from build123d import *

# Parameters (mm, degrees)
SKETCH_1_R      = 18.5
SKETCH_1_R_2    = 5
SKETCH_1_R_3    = 2
SKETCH_1_R_4    = 2.08
EXTRUDE_1_DEPTH = 2


with BuildPart() as part:
    # 草图1 → 凸台-拉伸1 (new body)
    with BuildSketch(Plane.XY):
        Circle(SKETCH_1_R)
        Circle(SKETCH_1_R_2, mode=Mode.SUBTRACT)
        with Locations((0, 15)):
            Circle(SKETCH_1_R_3, mode=Mode.SUBTRACT)
        with Locations((12.990381057, -7.5)):
            Circle(SKETCH_1_R_3, mode=Mode.SUBTRACT)
        with Locations((-12.990381057, -7.5)):
            Circle(SKETCH_1_R_3, mode=Mode.SUBTRACT)
        with Locations((-12.36258754, 7.137543244)):
            Circle(SKETCH_1_R_4, mode=Mode.SUBTRACT)
        with Locations((12.36258754, 7.137543244)):
            Circle(SKETCH_1_R_4, mode=Mode.SUBTRACT)
        with Locations((0, -14.275086489)):
            Circle(SKETCH_1_R_4, mode=Mode.SUBTRACT)
    extrude(amount=EXTRUDE_1_DEPTH)


solid = part.part
Geometry: final body of the model. Coordinates: model frame, mm. Give positions to 0.01 mm unless a question says otherwise; leave off trailing zeros. Order: outer loops, then holes, each group sorted by start corner. A loop starts at its lowest first (then second) coordinate and runs counter-clockwise, first axis right, second up. Notation, with made-up numbers: (65.25, 26) -> (84.25, 26) arc R28 cw to (84.25, 64) -> close; hole circle Ø8 at (71, 83). An arc over 180 degrees is marked (long way). Answer as a JSON object with one key per item and string values.
Q1. Section D-D (y = -6). Output: boundary loops of the cut face in (x, z).
Entries:
{"outline": "(-17.5, 0) -> (-14.31, 0) -> (-14.31, 2) -> (-17.5, 2) -> close; (-11.67, 0) -> (11.67, 0) -> (11.67, 2) -> (-11.67, 2) -> close; (14.31, 0) -> (17.5, 0) -> (17.5, 2) -> (14.31, 2) -> close"}
Q2. Material intervals for probe 1 along Y at (x, z) = (0, 1.2); probe 2 along X at (y, z) = (-8, 1.05); probe 3 along X at (y, z) = (-9, 1.55), sorted ascending.
Entries:
{"probe 1": "y = -18.5 to -16.36, -12.2 to -5, 5 to 13, 17 to 18.5", "probe 2": "x = -16.68 to -14.93, -11.05 to 11.05, 14.93 to 16.68", "probe 3": "x = -16.16 to -14.31, -11.67 to 11.67, 14.31 to 16.16"}
Q3. Section C-C (z = 0.4). Output: boundary loops of the cut face in (x, y), plus the area to 3 significant figures.
Entries:
{"outline": "circle Ø37 at (0, 0); hole circle Ø4 at (-12.99, -7.5); hole circle Ø4.16 at (-12.36, 7.14); hole circle Ø10 at (0, 0); hole circle Ø4.16 at (0, -14.28); hole circle Ø4 at (0, 15); hole circle Ø4.16 at (12.36, 7.14); hole circle Ø4 at (12.99, -7.5)", "area": "918 mm^2"}
Q4. Section B-B (y = 0). Output: boundary loops of the cut face in (x, z).
Entries:
{"outline": "(-18.5, 0) -> (-5, 0) -> (-5, 2) -> (-18.5, 2) -> close; (5, 0) -> (18.5, 0) -> (18.5, 2) -> (5, 2) -> close"}
Q5. Section A-A (x = 0). Output: boundary loops of the cut face in (y, z), plus the area to 3 significant figures.
Entries:
{"outline": "(-18.5, 0) -> (-16.36, 0) -> (-16.36, 2) -> (-18.5, 2) -> close; (-12.2, 0) -> (-5, 0) -> (-5, 2) -> (-12.2, 2) -> close; (5, 0) -> (13, 0) -> (13, 2) -> (5, 2) -> close; (17, 0) -> (18.5, 0) -> (18.5, 2) -> (17, 2) -> close", "area": "37.7 mm^2"}
Q6. Draft query along X for faces 1 (the cylindrical face through (-4.01, -18.06, 0.99)), 2 (the flat face through (4, -4, 0)), 3 (the cylindrical face through (-1.08, -4.88, 0.99)). Return one class per face: released by +X, released by -X, zero draft, split by the parting line, or undercut.
Entries:
{"face 1": "split by the parting line", "face 2": "zero draft", "face 3": "undercut"}
